Design review of the part built by this model. Coordinates are the model's own, in mm. A direction names the side the tool comes from. Coordinates: 2 decimals unless noted, no trailing zeros. Loops run counter-clockwise (first coordinate to the right, second up) from the corner with the lowest first, then second, coordinate; pieces in that order, holes last.
Q1. Machinability: for faces 4 (the face through (1.9, -9, 5)), 5 (the face through (-1.9, 3, -3)), 6 (the face through (-4.9, 2, 7)), which of the approach directions +Z, -Z, +X, -X, +Y, -Y give a long, thin tool a straight path to every point of the face, cutting with its end or side? Answer none if there is none.
Q2. Draft analysis for pull direction Z (two halves, no side actions). For faces 1 (the face through (1.9, 3, -3)), 2 (the face through (4.9, 2, 7)), 3 (the face through (-3.421, 6.039, 7.876)), state which applies: released by +Z, released by -Z, zero draft, split by the parting line, or undercut.
Q3. Add section C-C on x = -2.75. Give the boundary of the cut face in (y, z) (3 decimals).
Q4. Add section A-A on y = 0. Give the boundary of the cut face in (x, z) (3 decimals), and give its area (3 significant figures).
Q5. Wall thickness on probe 1 along Y at (x, z) = (-3.1, 0) (3 decimals); probe 2 along X at (y, z) = (4.75, 2); probe 3 along Y at (x, z) = (-0.5, -6.75): over which ranges is each line inside the solid? List them lowest first.
Q6. Add section D-D on y = 8. Give the boundary of the cut face in (x, z).
Q7. For P1, Ø2, axis at x = 2.5, y = -8, coming from the +Z side; P2, Ø10.5, axis at y = 0, z = 0, coming from the -X side; P3, Ø1.5, axis at x = 3, y = 9.5, coming from the -Z side; P4, Ø4, axis at y = 1.5, z = -0.5, coming from the +X side, all flat-tipped, find the tip position at first contact; note any pin that passes through.
```python
from build123d import *

# Parameters (mm, degrees)
F_8_1_8_1_DURCHMESSER_BOHRUNG1_D = 8.1


with BuildPart() as part:
    # Skizze1 → Rotation1 (revolve)
    with BuildSketch(Plane.XY, mode=Mode.PRIVATE) as rotation1_sk:
        Polygon((0, 0), (0, 12), (1.9, 12), (1.9, 9.925), (4.9, 9.925), (4.9, 7), (1.9, 7), (1.9, 0), align=None)
    rotation1 = revolve(rotation1_sk.sketch.rotate(Axis((0, 0, 0), (-1, 0, 0)), 90), axis=Axis((0, 0, 0), (-1, 0, 0)))

    # Ø8.1 (8.1) Durchmesser Bohrung1 (through all)
    with Locations(Plane.ZY):
        with Locations((0, 0)):
            f_8_1_8_1_durchmesser_bohrung1 = Hole(F_8_1_8_1_DURCHMESSER_BOHRUNG1_D / 2)

    # Spiegeln1: Rotation1, Ø8.1 (8.1) Durchmesser Bohrung1 across plane
    add(rotation1.mirror(Plane(origin=(0, 0, 0), x_dir=(0, 0, 1), z_dir=(1, 0, 0))))
    add(f_8_1_8_1_durchmesser_bohrung1.mirror(Plane(origin=(0, 0, 0), x_dir=(0, 0, 1), z_dir=(1, 0, 0))), mode=Mode.SUBTRACT)


solid = part.part
```
Entries:
1. face 4: +X
1. face 5: -X
1. face 6: +Z, -Z, -X, +Y, -Y
2. face 1: undercut
2. face 2: zero draft
2. face 3: split by the parting line
3. outline: circle Ø19.85 at (0, 0); hole circle Ø14 at (0, 0)
4. outline: (-4.9, -9.925) - (-1.9, -9.925) - (-1.9, -12) - (1.9, -12) - (1.9, -9.925) - (4.9, -9.925) - (4.9, -7) - (1.9, -7) - (1.9, -4.05) - (-1.9, -4.05) - (-1.9, -7) - (-4.9, -7) - close; (-4.9, 7) - (-1.9, 7) - (-1.9, 4.05) - (1.9, 4.05) - (1.9, 7) - (4.9, 7) - (4.9, 9.925) - (1.9, 9.925) - (1.9, 12) - (-1.9, 12) - (-1.9, 9.925) - (-4.9, 9.925) - close
4. area: 95.5 mm2
5. probe 1: y = -9.925 to -7, 7 to 9.925
5. probe 2: x = -1.9 to 1.9
5. probe 3: y = -9.92 to 9.92
6. outline: (-4.9, -5.87) - (-1.9, -5.87) - (-1.9, -8.94) - (1.9, -8.94) - (1.9, -5.87) - (4.9, -5.87) - (4.9, 5.87) - (1.9, 5.87) - (1.9, 8.94) - (-1.9, 8.94) - (-1.9, 5.87) - (-4.9, 5.87) - close
7. P1: stops at z = 9.6
7. P2: stops at x = -1.9
7. P3: stops at z = -4.68
7. P4: passes through
